from build123d import *

# Parameters (mm, degrees)
CONG_1_R = 1


with BuildPart() as part:
    # Esquisse1 → Base-Révolution (revolve)
    with BuildSketch(Plane.XY, mode=Mode.PRIVATE) as base_r_volution_sk:
        with BuildLine():
            Line((0, 5), (14, 5))
            Line((14, 5), (14, 8.5))
            Line((14, 8.5), (12.848076211, 8.5))
            ThreePointArc((12.848076211, 8.5), (10.25, 7), (7.651923789, 8.5))
            Line((7.651923789, 8.5), (6.348076211, 8.5))
            ThreePointArc((6.348076211, 8.5), (3.75, 7), (1.151923789, 8.5))
            Line((1.151923789, 8.5), (0, 8.5))
            Line((0, 8.5), (0, 5))
        make_face()
    revolve(base_r_volution_sk.sketch.rotate(Axis((0, 0, 0), (1, 0, 0)), 90), axis=Axis((0, 0, 0), (1, 0, 0)))

    # Congé1
    cong_1_edges = [part.edges().sort_by_distance(p)[0] for p in [
        (14, 0, -5),
        (0, 0, -5),
    ]]
    fillet(cong_1_edges, radius=CONG_1_R)


solid = part.part
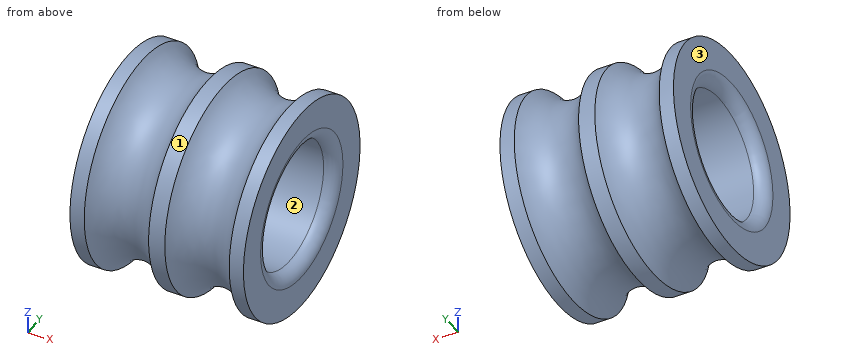
Verification items for the finished model (mm, model axes). Face numbers are marked on the shaded views. Coordinates: 2 decimals unless noted, no trailing zeros. Order: outer loops, then holes, each group sorted by start corner. A loop starts at its lowest first (then second) coordinate and runs counter-clockwise, first axis right, second up. Notation, with made-up numbers: (85, 77.5) -> (131, 77.5) arc R26 ccw to (131, 96.5) -> close; hole circle Ø4 at (29, 81.5). An arc over 180 degrees is marked (long way). Use CSV: the item, a comma, the result in double quotes. Start each with the question number.
Q1. Section check A-A, the plane z = 0. Record the cut outline in (x, y), and give its area (3 significant figures).
Q2. Depth check by flat-ended pin: P1, Ø5, axis at x = 9.5, z = 2.5, coming from the -Y side; P2, Ø4, axis at x = 6, z = -4.5, coming from the -Y side; P3, Ø1, axis at x = 3, y = 0, coming from the -Z side. Enter the tip coordinate at first touch or a pass-through.
Q3. Section check D-D, the plane z = -7.25. Give the number of separate pieces and of enclosed holes in the cut face, and give its area (3 significant figures).
Q4. Thickness scan on line 1 along X through (y, z) = (7, 3.75); line 2 along X through (y, z) = (-6.75, 5); line 3 along Z through (x, y) = (4.5, -1.75). Record the ranges inside material, lowest first.
Q5. Section check C-C, the plane x = 8. Record the cut outline in (y, z), and give its area (3 significant figures).
Q6. Draft check along Y on the marked faces 1, 2 and 3. Enter one of: +Y half, -Y half, draft (parallel to the pull), parting line (faces both ways), or undercut.
Returned:
1,outline,"(0, -8.5) -> (1.15, -8.5) arc R3 cw to (6.35, -8.5) -> (7.65, -8.5) arc R3 cw to (12.85, -8.5) -> (14, -8.5) -> (14, -6) arc R1 ccw to (13, -5) -> (1, -5) arc R1 ccw to (0, -6) -> close; (0, 6) arc R1 ccw to (1, 5) -> (13, 5) arc R1 ccw to (14, 6) -> (14, 8.5) -> (12.85, 8.5) arc R3 cw to (7.65, 8.5) -> (6.35, 8.5) arc R3 cw to (1.15, 8.5) -> (0, 8.5) -> close"
1,area,"75.0 mm^2"
2,P1,"stops at y = -8.46"
2,P2,"stops at y = -8.11"
2,P3,"stops at z = -7.27"
3,separate pieces,"3"
3,enclosed holes,"0"
3,area,"60.0 mm^2"
4,line 1,"x = 0 to 1.57, 5.93 to 8.07, 12.43 to 14"
4,line 2,"x = 0 to 1.21, 6.29 to 7.71, 12.79 to 14"
4,line 3,"z = -6.88 to -4.68, 4.68 to 6.88"
5,outline,"circle Ø16.03 at (0, 0); hole circle Ø10 at (0, 0)"
5,area,"123 mm^2"
6,face 1,"parting line"
6,face 2,"undercut"
6,face 3,"draft"
